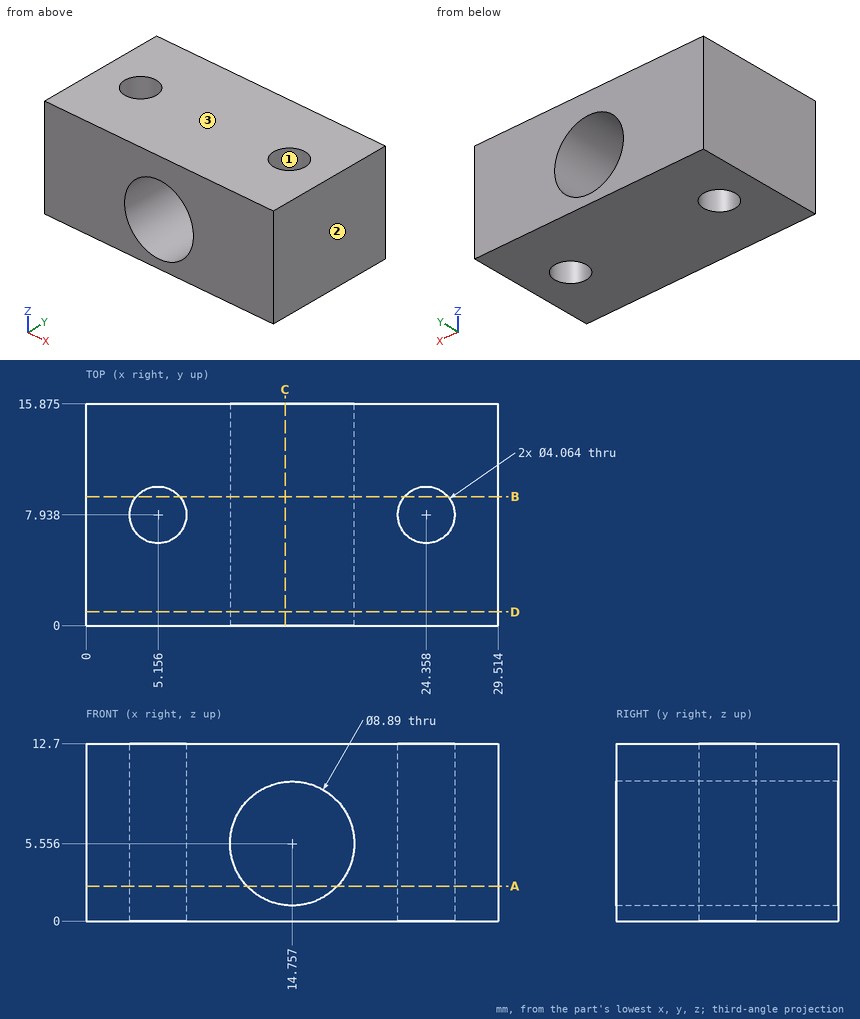
Source: three-view drawing plus pictorial views. Frame: mm from the lowest corner of the part. Round coordinates to 2 decimals unless told otherwise and drop trailing zeros. Write each loop counter-clockwise with the first axis right and the second up, starting at its lowest first coordinate (ties: lowest second). Pieces come first, ordered by that corner, then holes. Notation, with made-up numbers: M 48,-36 L 68,-36 A32 cw 68,-8 Z; hole C 72.5,25.25 d7. An arc over 180 degrees is marked long. Use CSV: the item, a comma, the result in double quotes. Start each with the question number.
Q1. Cut plane C-C on x = 14.25. Output: boundary loops of the cut face in (y, z) (1 decimal).
Q2. Cut plane D-D on y = 1. Output: boundary loops of the cut face in (x, z) (1 decimal).
Q3. Cut plane B-B on y = 9.25. Output: boundary loops of the cut face in (x, z) (1 decimal).
Q4. Line query: line 1 (X direction, y = 8, z = 12.25) (1 decimal); line 2 (X direction, y = 9.75, z = 4.5) (1 decimal); line 3 (Z direction, x = 12, y = 15.25) (1 decimal). Output: solid intervals per line, ascending. Write a range as from..to.
Q5. Pull-direction query (X, two-part tool) for the marked faces 1, 2 and 3; classes: +X half, -X half, draft (parallel to the pull), parting line (faces both ways), or undercut.
Q6. Cut plane A-A on z = 2.5. Output: boundary loops of the cut face in (x, y) (1 decimal), plus the area to 3 significant figures.
Results found:
1,outline,"M 0,0 L 15.9,0 L 15.9,1.1 L 0,1.1 Z; M 0,10 L 15.9,10 L 15.9,12.7 L 0,12.7 Z"
2,outline,"M 0,0 L 29.5,0 L 29.5,12.7 L 0,12.7 Z; hole C 14.8,5.6 d8.9"
3,outline,"M 0,0 L 3.6,0 L 3.6,12.7 L 0,12.7 Z; M 6.7,0 L 22.8,0 L 22.8,12.7 L 6.7,12.7 Z; M 25.9,0 L 29.5,0 L 29.5,12.7 L 25.9,12.7 Z; hole C 14.8,5.6 d8.9"
4,line 1,"0..3.1, 7.2..22.3, 26.4..29.5"
4,line 2,"0..4.2, 6.1..10.4, 19.1..23.4, 25.3..29.5"
4,line 3,"0..2.1, 9..12.7"
5,face 1,"undercut"
5,face 2,"+X half"
5,face 3,"draft"
6,outline,"M 0,0 L 11.5,0 L 11.5,15.9 L 0,15.9 Z; M 18,0 L 29.5,0 L 29.5,15.9 L 18,15.9 Z; hole C 5.2,7.9 d4.1; hole C 24.4,7.9 d4.1"
6,area,"340 mm^2"
